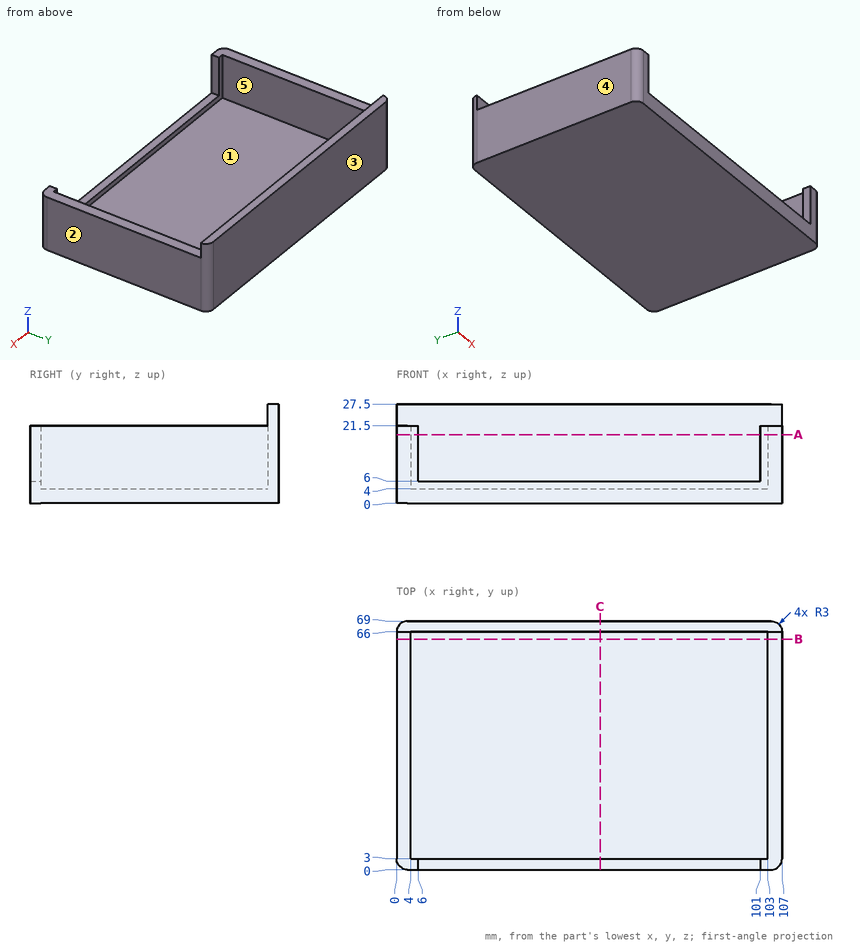
Design review of the part shown in the three views and the two pictorial views. Dimensions are in mm from the part's minimum x, y and z. A direction names the side the tool comes from. Coordinates: 2 decimals unless noted, no trailing zeros. Order: outer loops, then holes, each group sorted by start corner. A loop starts at its lowest first (then second) coordinate and runs counter-clockwise, first axis right, second up.
1) Wall thickness on line 1 along X through (y, z) = (43, 4.5); line 2 along Y through (x, z) = (98, 5.5); line 3 along Y through (x, z) = (10.5, 17): over which ranges is each line inside the solid? List them lowest first.
2) Take a section at A-A, the plane z = 19. Give the boundary of the cut face in (x, y).
3) Take a section at B-B, the plane y = 64. Give the boundary of the cut face in (x, z), and give its area (3 significant figures).
4) Take a section at C-C, the plane x = 56.5. Give the boundary of the cut face in (y, z), and give its area (4 significant figures).
5) Clearance check with flat-ended pins moving along their axes: pin 1 (2.5 mm diameter, centred on y = 1, z = 14.5, fed in from -X); pin 2 (3 mm diameter, centred on x = 61.5, z = 10, fed in from -Y); pin 3 (19 mm diameter, centred on x = 59, y = 46.5, fed in from +Z); pin 4 (2 mm diameter, centred on x = 67, y = 60, fed in from -Z). State where each tip first meets the part, or that it passes through.
6) Mouldability with a two-part tool opening along Y and no side actions: class the marked faces 3, 4 and 5 as +Y half, -Y half, draft (parallel to the pull), parting line (faces both ways), or undercut.
7) For the marked faces 1 and 2, list the 3-axis set-ups (+Z, -Z, +X, -X, +Y, -Y) from which the entire face can be reached by the end or side of a thin tool; tool diameter is ignored.
Returned:
1. line 1: x = 0 to 4, 103 to 107
1. line 2: y = 0 to 3, 66 to 69
1. line 3: y = 66 to 69
2. outline: (0, 3) arc R3 ccw to (3, 0) - (6, 0) - (6, 3) - (4, 3) - (4, 66) - (103, 66) - (103, 3) - (101, 3) - (101, 0) - (104, 0) arc R3 ccw to (107, 3) - (107, 66) arc R3 ccw to (104, 69) - (3, 69) arc R3 ccw to (0, 66) - close
3. outline: (0, 0) - (107, 0) - (107, 21.5) - (103, 21.5) - (103, 4) - (4, 4) - (4, 21.5) - (0, 21.5) - close
3. area: 568 mm2
4. outline: (0, 0) - (69, 0) - (69, 27.5) - (66, 27.5) - (66, 4) - (3, 4) - (3, 6) - (0, 6) - close
4. area: 352.5 mm2
5. pin 1: stops at x = 0.1
5. pin 2: stops at y = 66
5. pin 3: stops at z = 4
5. pin 4: stops at z = 0
6. face 3: +Y half
6. face 4: draft
6. face 5: undercut
7. face 1: +Z
7. face 2: +Z, -Z, +X, +Y, -Y
